from build123d import *

# Parameters (mm, degrees)
BOSS_EXTRUDE1_START = 4.5
SKETCH2_R           = 0.25
BOSS_EXTRUDE1_DEPTH = 2
BOSS_EXTRUDE2_START = -6.5
SKETCH2_2_R         = 0.25
BOSS_EXTRUDE2_DEPTH = 2
FILLET1_R           = 2
FILLET2_R           = 2
FILLET3_R           = 1
FILLET4_R           = 1


with BuildPart() as part:
    # Sketch1 → Revolve1 (revolve)
    with BuildSketch(Plane.XY, mode=Mode.PRIVATE) as revolve1_sk:
        Polygon((-1.75, 8.7), (-1.75, -8.7), (-1.7, -8.7), (-1.7, -9.5), (-1.625, -9.5), (-1.625, -10), (-1.5, -10), (-1.5, 10), (-1.625, 10), (-1.625, 9.5), (-1.7, 9.5), (-1.7, 8.7), align=None)
    revolve(revolve1_sk.sketch.rotate(Axis((-1.5, 10, 0), (0, -1, 0)), 270), axis=Axis((-1.5, 10, 0), (0, -1, 0)))

    # Sketch2 → Boss-Extrude1 (add)
    with BuildSketch(Plane(origin=(0, 0, 0), x_dir=(1, 0, 0), z_dir=(0, 1, 0)).offset(BOSS_EXTRUDE1_START)):
        with BuildLine():
            Line((-1.212744122, 0.216988619), (0.334063036, -1.830719917))
            Line((0.334063036, -1.830719917), (4.334063036, -1.830719917))
            Line((4.334063036, -1.830719917), (7.809461076, 0.794541672))
            Line((7.809461076, 0.794541672), (9.31, 0))
            Line((9.31, 0), (9.012661236, -0.561541836))
            Line((9.012661236, -0.561541836), (7.952156278, 0))
            Line((7.952156278, 0), (4.575438683, -2.550719917))
            Line((4.575438683, -2.550719917), (-0.024391576, -2.550719917))
            Line((-0.024391576, -2.550719917), (-1.787255878, -0.216988619))
            ThreePointArc((-1.787255878, -0.216988619), (-1.716988619, 0.287255878), (-1.212744122, 0.216988619))
        make_face()
        with Locations(Location((-1.5, 0, 0), (0, 0, 270))):
            Circle(SKETCH2_R, mode=Mode.SUBTRACT)
    extrude(amount=BOSS_EXTRUDE1_DEPTH)

    # Sketch2_2 → Boss-Extrude2 (add)
    with BuildSketch(Plane(origin=(0, 0, 0), x_dir=(1, 0, 0), z_dir=(0, 1, 0)).offset(BOSS_EXTRUDE2_START)):
        with BuildLine():
            Line((-1.212744122, 0.216988619), (0.334063036, -1.830719917))
            Line((0.334063036, -1.830719917), (4.334063036, -1.830719917))
            Line((4.334063036, -1.830719917), (7.809461076, 0.794541672))
            Line((7.809461076, 0.794541672), (9.31, 0))
            Line((9.31, 0), (9.012661236, -0.561541836))
            Line((9.012661236, -0.561541836), (7.952156278, 0))
            Line((7.952156278, 0), (4.575438683, -2.550719917))
            Line((4.575438683, -2.550719917), (-0.024391576, -2.550719917))
            Line((-0.024391576, -2.550719917), (-1.787255878, -0.216988619))
            ThreePointArc((-1.787255878, -0.216988619), (-1.716988619, 0.287255878), (-1.212744122, 0.216988619))
        make_face()
        with Locations(Location((-1.5, 0, 0), (0, 0, 270))):
            Circle(SKETCH2_2_R, mode=Mode.SUBTRACT)
    extrude(amount=BOSS_EXTRUDE2_DEPTH)

    # Fillet1
    fillet1_edges = [part.edges().sort_by_distance(p)[0] for p in [
        (4.334063036, 5.5, 1.830719917),
        (0.334063036, 5.5, 1.830719917),
        (4.334063036, -5.5, 1.830719917),
        (0.334063036, -5.5, 1.830719917),
    ]]
    fillet(fillet1_edges, radius=FILLET1_R)

    # Fillet2
    fillet2_edges = [part.edges().sort_by_distance(p)[0] for p in [
        (-0.024391576, 5.5, 2.550719917),
        (4.575438683, 5.5, 2.550719917),
        (-0.024391576, -5.5, 2.550719917),
        (4.575438683, -5.5, 2.550719917),
    ]]
    fillet(fillet2_edges, radius=FILLET2_R)

    # Fillet3
    fillet3_edges = [part.edges().sort_by_distance(p)[0] for p in [
        (7.809461076, 5.5, -0.794541672),
        (7.809461076, -5.5, -0.794541672),
    ]]
    fillet(fillet3_edges, radius=FILLET3_R)

    # Fillet4
    fillet4_edges = [part.edges().sort_by_distance(p)[0] for p in [
        (7.952156278, 5.5, 0),
        (7.952156278, -5.5, 0),
    ]]
    fillet(fillet4_edges, radius=FILLET4_R)


solid = part.part
Source: CAD feature listing. Evaluate the final solid. Frame: model axes, mm. A direction names the side the tool comes from. Coordinates: 2 decimals unless noted, no trailing zeros. Loops run counter-clockwise (first coordinate to the right, second up) from the corner with the lowest first, then second, coordinate; pieces in that order, holes last. Notation, with made-up numbers: (17, 63) - (63, 63) arc R8 cw to (63, 73) - close; hole circle Ø2 at (50, 55.25). An arc over 180 degrees is marked (long way). Return JSON: item names as keys, results as strings.
Q1. Material intervals for line 1 along Y through (x, z) = (-0.25, 1.4); line 2 along Z through (x, y) = (1.5, -5); line 3 along X through (y, z) = (5.25, -0.3), sorted ascending.
Results:
{"line 1": "-6.5 to -4.5, 4.5 to 6.5", "line 2": "1.83 to 2.55", "line 3": "-1.7 to -1.3, 7.15 to 8.74"}
Q2. Section B-B, the plane y = -6. Return loops of the section in (x, z), plus the area to 3 significant figures.
Results:
{"outline": "(-1.79, 0.22) arc R0.36 ccw to (-1.21, -0.22) - (-0.27, 1.04) arc R2 cw to (1.33, 1.83) - (3.66, 1.83) arc R2 cw to (4.87, 1.43) - (7.3, -0.41) arc R1 ccw to (8.37, -0.5) - (9.31, 0) - (9.01, 0.56) - (8.51, 0.3) arc R1 cw to (7.44, 0.38) - (5.11, 2.15) arc R2 ccw to (3.9, 2.55) - (0.97, 2.55) arc R2 ccw to (-0.62, 1.76) - close", "area": "9.29 mm2"}
Q3. Section D-D, the plane y = 1. Return loops of the section in (x, z).
Results:
{"outline": "circle Ø0.5 at (-1.5, 0)"}
Q4. Mould query, pull axis Y, two halves, no side actions, for faces 3 (the flat face through (4, 4.5, 2)), 4 (the cylindrical face through (0.068, -5.486, 2.335)), 5 (the flat face through (4, 6.5, 2)). Classes: released by +Y, released by -Y, zero draft, split by the parting line, or undercut.
Results:
{"face 3": "undercut", "face 4": "zero draft", "face 5": "released by +Y"}
Q5. Section C-C, the plane x = 8.75. Return loops of the section in (y, z).
Results:
{"outline": "(-6.5, -0.3) - (-4.5, -0.3) - (-4.5, 0.42) - (-6.5, 0.42) - close; (4.5, -0.3) - (6.5, -0.3) - (6.5, 0.42) - (4.5, 0.42) - close"}
Q6. Contact query for flat-ended pins moving along their axis: P1, Ø1.6, axis at x = 4.5, z = 1.5, coming from the +Y side; P2, Ø1.6, axis at x = 2.5, y = -5.5, coming from the -Z side. Output: stop coordinate, or through.
Results:
{"P1": "y = 6.5", "P2": "z = 1.83"}
Q7. Access query for faces 1 (the cylindrical face through (7.975, -5.486, 0.184)), 2 (the flat face through (6.07, -5.51, 0.52)). Directions: +Z, -Z, +X, -X, +Y, -Y. A direction counts if a zero-diameter tool reaches every point of the face in a straight line with its end or side. Return the directions, or none.
Results:
{"face 1": "+Z, +Y, -Y", "face 2": "-Z, +Y, -Y"}
Q8. Section A-A, the plane x = 0.25. Return loops of the section in (y, z), plus the area to 3 significant figures.
Results:
{"outline": "(-6.5, 1.51) - (-4.5, 1.51) - (-4.5, 2.42) - (-6.5, 2.42) - close; (4.5, 1.51) - (6.5, 1.51) - (6.5, 2.42) - (4.5, 2.42) - close", "area": "3.61 mm2"}
